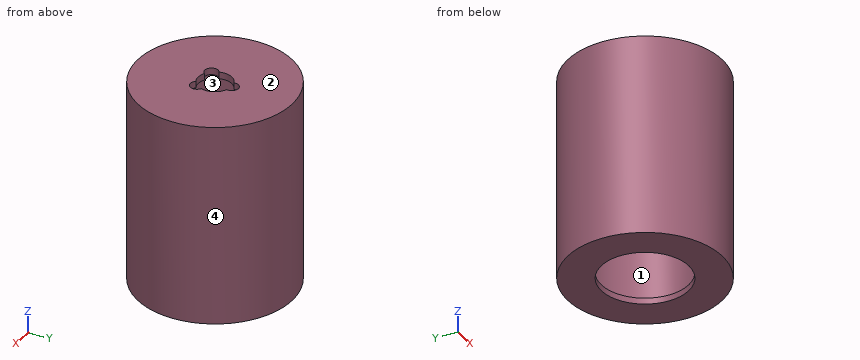
from build123d import *

# Parameters (mm, degrees)
SKETCH1_W          = 3.5
SKETCH1_H          = 5
SKETCH1_W_2        = 27.3
SKETCH1_W_3        = 25.5
CUT_EXTRUDE1_DEPTH = 2
SKETCH3_5_R        = 17
CUT_EXTRUDE2_DEPTH = 1
CUT_EXTRUDE3_START = -2
SKETCH5_R          = 5
SKETCH5_R_2        = 2
CUT_EXTRUDE3_DEPTH = 2


with BuildPart() as part:
    # Sketch1 → Revolve1 (revolve)
    with BuildSketch(Plane(origin=(0, 0, 0), x_dir=(0, 0, -1), z_dir=(1, 0, 0)), mode=Mode.PRIVATE) as revolve1_sk:
        Polygon((-59.8, 18), (-59.8, 5), (-57.8, 5), (-57.8, 17), (-30.8, 17), (-30.8, 18), (-34.3, 18), align=None)
        with Locations((-32.55, 20.5)):
            Rectangle(SKETCH1_W, SKETCH1_H)
        with Locations((-29.05, 20.5)):
            Rectangle(SKETCH1_W, SKETCH1_H)
        Polygon((-30.8, 18), (-30.8, 17), (-1.8, 17), (-1.8, 13), (0, 13), (0, 18), (-27.3, 18), align=None)
        with Locations((-13.65, 20.5)):
            Rectangle(SKETCH1_W_2, SKETCH1_H)
        with Locations((-47.05, 20.5)):
            Rectangle(SKETCH1_W_3, SKETCH1_H)
    revolve(revolve1_sk.sketch.rotate(Axis((0, 0, 1072.381477522), (0, 0, -1)), 90), axis=Axis((0, 0, 1072.381477522), (0, 0, -1)))

    # Sketch3 → Cut-Extrude1 (cut, symmetric)
    with BuildSketch(Plane.XY.offset(30.8)):
        with BuildLine():
            ThreePointArc((-6.566786752, 18.042098319), (0, -19.2), (6.566786752, 18.042098319))
            Line((6.566786752, 18.042098319), (7.592847182, 20.861176181))
            ThreePointArc((7.592847182, 20.861176181), (0, 22.2), (-7.592847182, 20.861176181))
            Line((-7.592847182, 20.861176181), (-6.566786752, 18.042098319))
        make_face()
        with BuildLine():
            add(Edge.make_bspline(
                [(-1, 19.972224976), (-1.837517439, 19.972224976), (-3.400688885, 17.606551444), (-4.505268868, 16.51808236)],
                knots=[0, 0, 0, 0, 1, 1, 1, 1], degree=3))
            Line((-1, 19.972224976), (1, 19.972224976))
            add(Edge.make_bspline(
                [(1, 19.972224976), (1.837517439, 19.972224976), (3.400688885, 17.606551444), (4.505268868, 16.51808236)],
                knots=[0, 0, 0, 0, 1, 1, 1, 1], degree=3))
            Line((4.505268868, 16.51808236), (4.683975969, 16.341981799))
            ThreePointArc((4.683975969, 16.341981799), (13.576221703, 10.231627645), (17, 0))
            ThreePointArc((17, 0), (-10.231627645, -13.576221703), (-4.683975969, 16.341981799))
            Line((-4.683975969, 16.341981799), (-4.505268868, 16.51808236))
        make_face(mode=Mode.SUBTRACT)
    extrude(amount=CUT_EXTRUDE1_DEPTH, both=True, mode=Mode.SUBTRACT)

    # Sketch3_5 → Cut-Extrude2 (cut, symmetric)
    with BuildSketch(Plane.XY.offset(30.8)):
        Circle(SKETCH3_5_R)
        with BuildLine():
            Line((1, 19.972224976), (-1, 19.972224976))
            add(Edge.make_bspline(
                [(-1, 19.972224976), (-1.837517439, 19.972224976), (-3.400688885, 17.606551444), (-4.505268868, 16.51808236)],
                knots=[0, 0, 0, 0, 1, 1, 1, 1], degree=3))
            Line((-4.505268868, 16.51808236), (-4.683975969, 16.341981799))
            ThreePointArc((-4.683975969, 16.341981799), (0, 17), (4.683975969, 16.341981799))
            Line((4.683975969, 16.341981799), (4.505268868, 16.51808236))
            add(Edge.make_bspline(
                [(1, 19.972224976), (1.837517439, 19.972224976), (3.400688885, 17.606551444), (4.505268868, 16.51808236)],
                knots=[0, 0, 0, 0, 1, 1, 1, 1], degree=3))
        make_face()
        with BuildLine():
            Line((7.592847182, 20.861176181), (6.566786752, 18.042098319))
            ThreePointArc((6.566786752, 18.042098319), (0, -19.2), (-6.566786752, 18.042098319))
            Line((-6.566786752, 18.042098319), (-7.592847182, 20.861176181))
            ThreePointArc((-7.592847182, 20.861176181), (-12.733396887, -18.185175383), (22.2, 0))
            ThreePointArc((22.2, 0), (18.185175383, 12.733396887), (7.592847182, 20.861176181))
        make_face()
    extrude(amount=CUT_EXTRUDE2_DEPTH, both=True, mode=Mode.SUBTRACT)

    # Sketch5 → Cut-Extrude3 (cut)
    with BuildSketch(Plane.XY.offset(59.8).offset(CUT_EXTRUDE3_START)):
        Circle(SKETCH5_R)
        with Locations((-3.830222216, -3.213938048)):
            Circle(SKETCH5_R_2)
        with Locations((0, 5)):
            Circle(SKETCH5_R_2)
        with Locations((3.830222216, -3.213938048)):
            Circle(SKETCH5_R_2)
    extrude(amount=CUT_EXTRUDE3_DEPTH, mode=Mode.SUBTRACT)


solid = part.part
Verification items for the finished model (mm, model axes). Face numbers are marked on the shaded views. Round coordinates to 2 decimals unless told otherwise and drop trailing zeros. Loops run counter-clockwise (first coordinate to the right, second up) from the corner with the lowest first, then second, coordinate; pieces in that order, holes last. Notation, with made-up numbers: (-9, 7.25) - (45, 7.25) arc R33 ccw to (45, 39.25) - close; hole circle Ø4 at (63.5, 63). An arc over 180 degrees is marked (long way). Use one line per item in the form item = value.
1. Section check D-D on z = 20. Record the cut outline in (x, y), and give its area (3 significant figures).
A:
outline = circle Ø46 at (0, 0); hole circle Ø34 at (0, 0)
area = 754 mm²
2. Section check C-C on y = -15. Record the cut outline in (x, z) (3 decimals).
A:
outline = (-17.436, 0) - (17.436, 0) - (17.436, 59.8) - (-17.436, 59.8) - close; hole (-16.366, 29.8) - (-11.985, 29.8) - (-11.985, 28.8) - (-8, 28.8) - (-8, 1.8) - (8, 1.8) - (8, 28.8) - (11.985, 28.8) - (11.985, 29.8) - (16.366, 29.8) - (16.366, 31.8) - (11.985, 31.8) - (11.985, 32.8) - (8, 32.8) - (8, 57.8) - (-8, 57.8) - (-8, 32.8) - (-11.985, 32.8) - (-11.985, 31.8) - (-16.366, 31.8) - close
3. Scan lines: probe 1 along Z at (x, y) = (18.5, 5.5); probe 2 along Z at (x, y) = (-5.5, 21); probe 3 along Y at (x, z) = (0, 13). Record each from-to range of solid material in increasing order.
A:
probe_1 = 0 to 29.8, 31.8 to 59.8
probe_2 = 0 to 28.8, 32.8 to 59.8
probe_3 = -23 to -17, 17 to 23
4. Draft check along X on the marked faces 1, 2, 3 and 4. Enter one of: pulls with the +X half, pulls with the -X half, needs draft (parallel to the pull), parting line crosses it, or undercut.
A:
face_1 = undercut
face_2 = needs draft
face_3 = undercut
face_4 = parting line crosses it
5. Gauge pin test, flat ends, axial feed: pin 1 Ø5 at (x, z) = (-15.5, 21) entering from -Y; pin 2 Ø12 at (x, z) = (-7.5, 11.5) entering from -Y; pin 3 Ø12 at (y, z) = (13.5, 21) entering from -X. Record the tip position at first contact, or that the pin passes through.
A:
pin_1 = -18.97
pin_2 = -22.95
pin_3 = -21.74
